Verification items for the finished model (mm, model axes). A direction names the side the tool comes from. Give positions to 0.01 mm unless a question says otherwise; leave off trailing zeros. Write each loop counter-clockwise with the first axis right and the second up, starting at its lowest first coordinate (ties: lowest second). Pieces come first, ordered by that corner, then holes. Notation, with made-up numbers: (71.5, -17.5) -> (96.5, -17.5) arc R17 cw to (96.5, 3.5) -> close; hole circle Ø1 at (-8.75, 27). An arc over 180 degrees is marked (long way). Use one line per item in the form item = value. Start each with the question number.
(1) Release check for a two-part mould opening along Y. For faces 1 (the face through (-28.542, 72.535, -29.604)), 2 (the face through (-25, 70, 25)), 3 (the face through (-1, 71.419, -3)) record: pulls with the +Y half, pulls with the -Y half, needs draft (parallel to the pull), parting line crosses it, or undercut.
(2) Scan lines: L1, parallel to Y at x = -16, z = 30; L2, parallel to X at y = -72, z = 0; L3, parallel to X at y = -72, z = 43. Record each from-to range of solid material in increasing order.
(3) Set-up check for faces 4 (the face through (1.32, 0.98, -29.97)), 5 (the face through (-5.9, -73, -0.8)), 6 (the face through (-30.22, -72.54, 28.32)): record each of +Z, -Z, +X, -X, +Y, -Y from which the full face is reachable in a straight line by a thin tool's end or side.
(4) Section check A-A, the plane z = 0. State how many separate pieces and enclosed holes the cut face has, plus the area to 3 significant figures.
(5) Depth check by flat-ended pin: pin 1 Ø3 at (x, z) = (30.76, 30.76) entering from -Y; pin 2 Ø1.5 at (y, z) = (-44.5, -4.5) entering from +X; pin 3 Ø9.5 at (x, z) = (0, 0) entering from -Y; pin 4 Ø6 at (y, z) = (34, 0) entering from -X. Enter the tip coordinate at first touch or a pass-through.
(6) Section check C-C, the plane y = 37. Record the cut outline in (x, z).
from build123d import *

# Parameters (mm, degrees)
SKETCH1_R               = 30
BOSS_EXTRUDE1_DEPTH     = 70
SKETCH2_R               = 60
BOSS_EXTRUDE2_DEPTH     = 5
FILLET1_R               = 2
FILLET5_R               = 3
SKETCH6_R               = 2.5
CUT_EXTRUDE1_DEPTH      = 169.0029762
CIRPATTERN1_COUNT       = 8
MIRROR1_COPY_1_SKETCH_R = 2.5
MIRROR1_COPY_1_DEPTH    = 169.0029762
MIRROR1_COPY_2_SKETCH_R = 2.5
MIRROR1_COPY_2_DEPTH    = 169.0029762
MIRROR1_COPY_3_SKETCH_R = 2.5
MIRROR1_COPY_3_DEPTH    = 169.0029762
MIRROR1_COPY_4_SKETCH_R = 2.5
MIRROR1_COPY_4_DEPTH    = 169.0029762
MIRROR1_COPY_5_SKETCH_R = 2.5
MIRROR1_COPY_5_DEPTH    = 169.0029762
MIRROR1_COPY_6_SKETCH_R = 2.5
MIRROR1_COPY_6_DEPTH    = 169.0029762
MIRROR1_COPY_7_SKETCH_R = 2.5
MIRROR1_COPY_7_DEPTH    = 169.0029762
FILLET1_OF_MIRROR1_R    = 2
FILLET5_OF_MIRROR1_R    = 3


with BuildPart() as part:
    # Sketch1 → Boss-Extrude1 (new, symmetric)
    with BuildSketch(Plane(origin=(0, 0, 0), x_dir=(1, 0, 0), z_dir=(0, 1, 0))):
        with Locations(Location((0, 0, 0), (0, 0, 270))):
            Circle(SKETCH1_R)
    extrude(amount=BOSS_EXTRUDE1_DEPTH, both=True)

    # Sketch2 → Boss-Extrude2 (add)
    with BuildSketch(Plane(origin=(0, 70, 0), x_dir=(1, 0, 0), z_dir=(0, 1, 0))):
        with Locations(Location((0, 0, 0), (0, 0, 270))):
            Circle(SKETCH2_R)
    boss_extrude2 = extrude(amount=BOSS_EXTRUDE2_DEPTH)

    # Fillet1
    fillet1_edges = [part.edges().sort_by_distance(p)[0] for p in [
        (0, 75, -60),
    ]]
    fillet(fillet1_edges, radius=FILLET1_R)

    # Fillet5
    fillet5_edges = [part.edges().sort_by_distance(p)[0] for p in [
        (0, 70, -60),
    ]]
    fillet(fillet5_edges, radius=FILLET5_R - 0.0001)  # a hair under: the kernel refuses the full size

    # Sketch5 → CBORE for #12 Binding Head Machine Screw1 (revolve, cut)
    with BuildSketch(Plane(origin=(0, 75, 0), x_dir=(0, 0, 1), z_dir=(1, 0, 0))):
        Polygon((0, 0), (0, 150), (2.8956, 150), (2.8956, 3.5814), (5.95376, 3.5814), (5.95376, 0.532828266), (6.58876, 0), align=None)
    cbore_for_12_binding_head_machine_screw = revolve(axis=Axis((0, 81.35, 0), (0, -1, 0)), mode=Mode.SUBTRACT)

    # Sketch6 → Cut-Extrude1 (cut, through all)
    with BuildSketch(Plane(origin=(0, 75, 0), x_dir=(1, 0, 0), z_dir=(0, 1, 0))):
        with Locations(Location((0, 43.5, 0), (0, 0, 270))):
            Circle(SKETCH6_R)
    cut_extrude1 = extrude(amount=-CUT_EXTRUDE1_DEPTH, mode=Mode.SUBTRACT)

    # CirPattern1: Cut-Extrude1 ×8 about axis
    cirpattern1_axis = Axis((0, 0, 0), (0, 1, 0))
    for i in range(1, CIRPATTERN1_COUNT):
        add(cut_extrude1.rotate(cirpattern1_axis, i * 360 / CIRPATTERN1_COUNT), mode=Mode.SUBTRACT)

    # Mirror1: Boss-Extrude2, CBORE for #12 Binding Head Machine Screw1, Cut-Extrude1 across plane
    add(boss_extrude2.mirror(Plane.ZX))
    add(cbore_for_12_binding_head_machine_screw.mirror(Plane.ZX), mode=Mode.SUBTRACT)
    add(cut_extrude1.mirror(Plane.ZX), mode=Mode.SUBTRACT)

    # Mirror1 copy 1 sketch → Mirror1 copy 1 (cut, through all)
    with BuildSketch(Plane(origin=(0, -75, 0), x_dir=(0.7071067811865476, 0, -0.7071067811865475), z_dir=(0, -1, 0))):
        with Locations((0, -43.5)):
            Circle(MIRROR1_COPY_1_SKETCH_R)
    extrude(amount=-MIRROR1_COPY_1_DEPTH, mode=Mode.SUBTRACT)

    # Mirror1 copy 2 sketch → Mirror1 copy 2 (cut, through all)
    with BuildSketch(Plane(origin=(0, -75, 0), x_dir=(0, 0, -1), z_dir=(0, -1, 0))):
        with Locations((0, -43.5)):
            Circle(MIRROR1_COPY_2_SKETCH_R)
    extrude(amount=-MIRROR1_COPY_2_DEPTH, mode=Mode.SUBTRACT)

    # Mirror1 copy 3 sketch → Mirror1 copy 3 (cut, through all)
    with BuildSketch(Plane(origin=(0, -75, 0), x_dir=(-0.7071067811865475, 0, -0.7071067811865476), z_dir=(0, -1, 0))):
        with Locations((0, -43.5)):
            Circle(MIRROR1_COPY_3_SKETCH_R)
    extrude(amount=-MIRROR1_COPY_3_DEPTH, mode=Mode.SUBTRACT)

    # Mirror1 copy 4 sketch → Mirror1 copy 4 (cut, through all)
    with BuildSketch(Plane(origin=(0, -75, 0), x_dir=(-1, 0, 0), z_dir=(0, -1, 0))):
        with Locations((0, -43.5)):
            Circle(MIRROR1_COPY_4_SKETCH_R)
    extrude(amount=-MIRROR1_COPY_4_DEPTH, mode=Mode.SUBTRACT)

    # Mirror1 copy 5 sketch → Mirror1 copy 5 (cut, through all)
    with BuildSketch(Plane(origin=(0, -75, 0), x_dir=(-0.7071067811865477, 0, 0.7071067811865475), z_dir=(0, -1, 0))):
        with Locations((0, -43.5)):
            Circle(MIRROR1_COPY_5_SKETCH_R)
    extrude(amount=-MIRROR1_COPY_5_DEPTH, mode=Mode.SUBTRACT)

    # Mirror1 copy 6 sketch → Mirror1 copy 6 (cut, through all)
    with BuildSketch(Plane(origin=(0, -75, 0), x_dir=(0, 0, 1), z_dir=(0, -1, 0))):
        with Locations((0, -43.5)):
            Circle(MIRROR1_COPY_6_SKETCH_R)
    extrude(amount=-MIRROR1_COPY_6_DEPTH, mode=Mode.SUBTRACT)

    # Mirror1 copy 7 sketch → Mirror1 copy 7 (cut, through all)
    with BuildSketch(Plane(origin=(0, -75, 0), x_dir=(0.7071067811865474, 0, 0.7071067811865477), z_dir=(0, -1, 0))):
        with Locations((0, -43.5)):
            Circle(MIRROR1_COPY_7_SKETCH_R)
    extrude(amount=-MIRROR1_COPY_7_DEPTH, mode=Mode.SUBTRACT)

    # Fillet1 of Mirror1
    fillet1_of_mirror1_edges = [part.edges().sort_by_distance(p)[0] for p in [
        (0, -75, -60),
    ]]
    fillet(fillet1_of_mirror1_edges, radius=FILLET1_OF_MIRROR1_R)

    # Fillet5 of Mirror1
    fillet5_of_mirror1_edges = [part.edges().sort_by_distance(p)[0] for p in [
        (0, -70, -60),
    ]]
    fillet(fillet5_of_mirror1_edges, radius=FILLET5_OF_MIRROR1_R - 0.0001)  # a hair under: the kernel refuses the full size


solid = part.part
Completed:
q1.face_1 = needs draft
q1.face_2 = undercut
q1.face_3 = pulls with the +Y half
q2.L1 = -75 to -70, 70 to 75
q2.L2 = -59.83 to -46, -41 to -5.95, 5.95 to 41, 46 to 59.83
q2.L3 = -41.6 to -2.45, 2.45 to 41.6
q3.face_4 = none
q3.face_5 = -Y
q3.face_6 = +Y, -Y
q4.separate_pieces = 6
q4.enclosed_holes = 0
q4.area = 8,580 mm²
q5.pin_1 = through
q5.pin_2 = 29.76
q5.pin_3 = -71.42
q5.pin_4 = -30
q6.outline = circle Ø60 at (0, 0); hole circle Ø5.79 at (0, 0)
